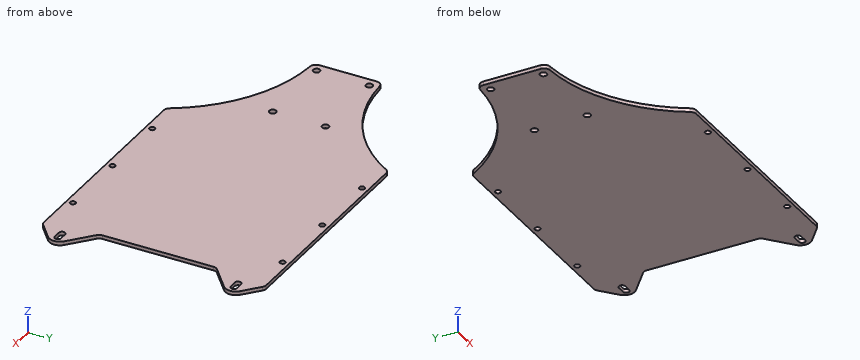
```python
from build123d import *

# Parameters (mm, degrees)
SKETCH_R   = 2.7
SKETCH_R_2 = 2.2
PAD_DEPTH  = 3
FILLET_R   = 5


with BuildPart() as part:
    # Sketch → Pad (new body)
    with BuildSketch(Plane.XY):
        with BuildLine():
            Line((-103.1, 27.65), (-103.1, 0))
            Line((-103.1, 0), (172.5, 0))
            Line((172.5, 46.548967), (172.5, 0))
            Line((172.5, 46.548967), (192.536791, 63.750663))
            ThreePointArc((192.536791, 63.750663), (195.5, 70.199983), (192.536817, 76.649314))
            Line((178.5, 88.7), (192.536817, 76.649314))
            Line((0, 88.7), (178.5, 88.7))
            ThreePointArc((-103.1, 27.65), (-43.385052, 44.386201), (0, 88.7))
        make_face()
        with Locations((-95.7, 21.05)):
            Circle(SKETCH_R, mode=Mode.SUBTRACT)
        with Locations((-32.2, 21.05)):
            Circle(SKETCH_R, mode=Mode.SUBTRACT)
        with Locations((86.25, 83.7)):
            Circle(SKETCH_R_2, mode=Mode.SUBTRACT)
        with Locations((28.75, 83.7)):
            Circle(SKETCH_R_2, mode=Mode.SUBTRACT)
        with Locations((143.75, 83.7)):
            Circle(SKETCH_R_2, mode=Mode.SUBTRACT)
        with BuildLine():
            ThreePointArc((184, 72.7), (181.5, 70.2), (184, 67.7))
            Line((184, 67.7), (190, 67.7))
            ThreePointArc((190, 67.7), (192.5, 70.2), (190, 72.7))
            Line((190, 72.7), (184, 72.7))
        make_face(mode=Mode.SUBTRACT)
    pad = extrude(amount=PAD_DEPTH)

    # Mirrored: Pad across XZ
    add(pad.mirror(Plane.XZ))

    # Fillet
    fillet_edges = [part.edges().sort_by_distance(p)[0] for p in [
        (178.5, -88.7, 1.5),
        (0, -88.7, 1.5),
        (-103.1, -27.65, 1.5),
        (192.536817, 76.649314, 1.5),
        (178.5, 88.7, 1.5),
        (0, 88.7, 1.5),
        (-103.1, 27.65, 1.5),
        (172.5, 46.548967, 1.5),
        (172.5, -46.548967, 1.5),
    ]]
    fillet(fillet_edges, radius=FILLET_R)


solid = part.part
```
Build history of the part. All positions in model axes, mm. Coordinates: 2 decimals unless noted, no trailing zeros. Order: outer loops, then holes, each group sorted by start corner. A loop starts at its lowest first (then second) coordinate and runs counter-clockwise, first axis right, second up.
Item 1: Saw through at B-B on x = -61. List the corners of the cut face in (y, z).
Filled in:
outline: (-35.81, 0) - (35.81, 0) - (35.81, 3) - (-35.81, 3) - close
Item 2: Drill centre lines: L1, parallel to X at y = -21.05, z = 1.3; L2, parallel to Y at x = 144.5, z = 0.2; L3, parallel to Y at x = -32.2, z = 1. Where is each one in solid material? Low to high.
Filled in:
L1: x = -103.1 to -98.4, -93 to -34.9, -29.5 to 172.5
L2: y = -88.7 to -85.77, -81.63 to 81.63, 85.77 to 88.7
L3: y = -51.89 to -23.75, -18.35 to 18.35, 23.75 to 51.89
Item 3: Saw through at A-A on z = 0.6. State how many separate pieces and enclosed holes the cut face has, then the cut area to 3 significant figures.
Filled in:
separate pieces: 1
enclosed holes: 12
area: 40,900 mm2
Item 4: Drop flat-ended pins along their axis: pin 1 Ø5 at (x, y) = (143.75, 83.7) entering from -Z; pin 2 Ø1 at (y, z) = (-40, 2.5) entering from -X; pin 3 Ø1.5 at (y, z) = (-15, 1.5) entering from +X; pin 4 Ø1.5 at (x, z) = (188, 1) entering from +Y. Give the stop position or say it passes through.
Filled in:
pin 1: stops at z = 0
pin 2: stops at x = -52.51
pin 3: stops at x = 172.5
pin 4: stops at y = 81.19
Item 5: Saw through at C-C on y = 54.5. List the corners of the cut face in (x, z).
Filled in:
outline: (-28.87, 0) - (181.76, 0) - (181.76, 3) - (-28.87, 3) - close
